```python
from build123d import *

# Parameters (mm, degrees)
SKETCH1_W           = 15
SKETCH1_H           = 15
BOSS_EXTRUDE1_DEPTH = 40
SKETCH2_W           = 9.8
SKETCH2_H           = 9.8
BOSS_EXTRUDE2_DEPTH = 28
SKETCH3_R           = 1.5
CUT_EXTRUDE1_DEPTH  = 69.822234779
SKETCH4_R           = 3.5
CUT_EXTRUDE2_DEPTH  = 6
SKETCH5_W           = 10.3
SKETCH5_H           = 10.3
CUT_EXTRUDE3_DEPTH  = 25
CUT_EXTRUDE8_DEPTH  = 10.3
SKETCH8_R           = 3.2
CUT_EXTRUDE10_DEPTH = 39.954720357


with BuildPart() as part:
    # Sketch1 → Boss-Extrude1 (new body)
    with BuildSketch(Plane(origin=(0, 0, 0), x_dir=(1, 0, 0), z_dir=(0, 1, 0))):
        Rectangle(SKETCH1_W, SKETCH1_H)
    extrude(amount=BOSS_EXTRUDE1_DEPTH)

    # Sketch2 → Boss-Extrude2 (add)
    with BuildSketch(Plane.XZ):
        Rectangle(SKETCH2_W, SKETCH2_H)
    extrude(amount=BOSS_EXTRUDE2_DEPTH)

    # Sketch3 → Cut-Extrude1 (cut, through all)
    with BuildSketch(Plane.XZ.offset(28)):
        with Locations(Location((0, 0, 0), (0, 0, 270))):
            Circle(SKETCH3_R)
    extrude(amount=-CUT_EXTRUDE1_DEPTH, mode=Mode.SUBTRACT)

    # Sketch4 → Cut-Extrude2 (cut)
    with BuildSketch(Plane.XZ.offset(28)):
        with Locations(Location((0, 0, 0), (0, 0, 270))):
            Circle(SKETCH4_R)
    extrude(amount=-CUT_EXTRUDE2_DEPTH, mode=Mode.SUBTRACT)

    # Sketch5 → Cut-Extrude3 (cut)
    with BuildSketch(Plane(origin=(0, 40, 0), x_dir=(1, 0, 0), z_dir=(0, 1, 0))):
        Rectangle(SKETCH5_W, SKETCH5_H)
    extrude(amount=-CUT_EXTRUDE3_DEPTH, mode=Mode.SUBTRACT)

    # Sketch6 → Cut-Extrude8 (cut)
    with BuildSketch(Plane.ZY.offset(-5.15)):
        Polygon((5.15, 15), (-4.95, 2.963288715), (-4.95, 15), align=None)
    extrude(amount=CUT_EXTRUDE8_DEPTH, mode=Mode.SUBTRACT)

    # Sketch8 → Cut-Extrude10 (cut, through all)
    with BuildSketch(Plane(origin=(0, 3.661758703, -4.36391409), x_dir=(-1, 0, 0), z_dir=(0, 0.6427876096865436, -0.7660444431189745))):
        with Locations(Location((0, 10.801022837, 0), (0, 0, 90))):
            Circle(SKETCH8_R)
    extrude(amount=-CUT_EXTRUDE10_DEPTH, mode=Mode.SUBTRACT)


solid = part.part
```
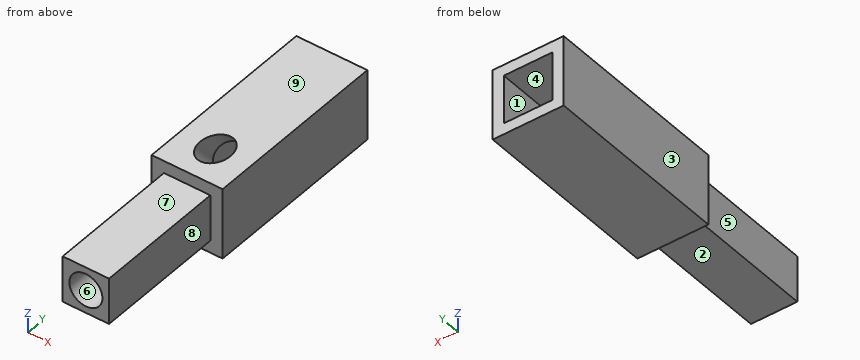
CAD build for the part. Positions are in the model's coordinates, mm. Face numbers are marked on the shaded views. A direction names the side the tool comes from. Coordinates: 2 decimals unless noted, no trailing zeros. Write each loop counter-clockwise with the first axis right and the second up, starting at its lowest first coordinate (ties: lowest second). Pieces come first, ordered by that corner, then holes. Notation, with made-up numbers: (7, 7.5) -> (16, 7.5) arc R29 cw to (16, 43.5) -> close; hole circle Ø9 at (17, -4). An arc over 180 degrees is marked (long way). Return JSON: item names as keys, results as strings. Group by question number.
Q1. Drill centre lines: line 1 (X direction, y = 27, z = 4); line 2 (X direction, y = -24.35, z = 0); line 3 (Z direction, x = 0, y = -3). Where is each one in solid material? Low to high.
Q2. Cut at B-B, the plane x = 0. Give the cut face in (y, z).
Q3. Cut at A-A, the plane z = 0. Give the cut face in (x, y), then the cut area to 3 significant figures.
Q4. Which spindle directions (+Z, -Z, +X, -X, +Y, -Y) get a long thin tool onto all of the face, cutting with end or side? Do the marked faces 5, 6, 7, 8 and 9. Say none if no direction does.
Q5. Flat gauge pins, fed straight in: pin 1 (3 mm diameter, centred on x = -1, y = -9, fed in from +Z); pin 2 (5 mm diameter, centred on x = 0, z = 0, fed in from -Y); pin 3 (8 mm diameter, centred on x = -2, y = -17, fed in from -Z). Where does each tip first touch, or does it go through?
Q6. Pull direction Z, two halves, no side cores. Call the marked faces 1, 2, 3 and 4: released by +Z, released by -Z, zero draft, split by the parting line, or undercut.
Q7. Cut at C-C, the plane y = -15.5. Give the cut face in (x, z), then the cut area to 3 significant figures.
Returned:
{
 "1": {"line 1": "x = -7.5 to -5.15, 5.15 to 7.5", "line 2": "x = -4.9 to -3.5, 3.5 to 4.9", "line 3": "z = -4.9 to -1.5, 1.5 to 4.9"},
 "2": {"outline": "(-28, -4.9) -> (0, -4.9) -> (0, -7.5) -> (40, -7.5) -> (40, -5.15) -> (15, -5.15) -> (15, -4.95) -> (2.96, -4.95) -> (7.07, -1.5) -> (-22, -1.5) -> (-22, -3.5) -> (-28, -3.5) -> close; (-28, 3.5) -> (-22, 3.5) -> (-22, 1.5) -> (8.66, 1.5) -> (3.63, 7.5) -> (0, 7.5) -> (0, 4.9) -> (-28, 4.9) -> close; (11.98, 7.5) -> (14.39, 4.64) -> (15, 5.15) -> (40, 5.15) -> (40, 7.5) -> close"},
 "3": {"outline": "(-7.5, 0) -> (-4.9, 0) -> (-4.9, -28) -> (-3.5, -28) -> (-3.5, -22) -> (-1.5, -22) -> (-1.5, 8.86) -> (-5.15, 8.86) -> (-5.15, 40) -> (-7.5, 40) -> close; (1.5, -22) -> (3.5, -22) -> (3.5, -28) -> (4.9, -28) -> (4.9, 0) -> (7.5, 0) -> (7.5, 40) -> (5.15, 40) -> (5.15, 8.86) -> (1.5, 8.86) -> close", "area": "419 mm2"},
 "4": {"face 5": "+Z, -Z, -X, -Y", "face 6": "-Y", "face 7": "+Z, +X, -X, -Y", "face 8": "+Z, -Z, +X, -Y", "face 9": "+Z, +X, -X, +Y, -Y"},
 "5": {"pin 1": "stops at z = 4.9", "pin 2": "stops at y = -22", "pin 3": "stops at z = -4.9"},
 "6": {"face 1": "undercut", "face 2": "released by -Z", "face 3": "zero draft", "face 4": "undercut"},
 "7": {"outline": "(-4.9, -4.9) -> (4.9, -4.9) -> (4.9, 4.9) -> (-4.9, 4.9) -> close; hole circle Ø3 at (0, 0)", "area": "89.0 mm2"}
}
